Read the model definition and answer for the solid it produces. Units are mm, in the model's axes. Face numbers are marked on the shaded views. Coordinates: 2 decimals unless noted, no trailing zeros. Order: outer loops, then holes, each group sorted by start corner. A loop starts at its lowest first (then second) coordinate and runs counter-clockwise, first axis right, second up. Notation, with made-up numbers: (-37.5, -0.75) - (-11.5, -0.75) arc R11 cw to (-11.5, 5.25) - close; hole circle Ø9 at (44.5, 49.5). An arc over 180 degrees is marked (long way). Use one line per item in the form item = value.
```python
from build123d import *

# Parameters (mm, degrees)
F0_R      = 15.875
F1_DEPTH  = 3.175
F1_FACE_R = 15.875
F2_DEPTH  = 25.4
F2_TAPER  = 15
F3_R      = 8.5725
F4_DEPTH  = 25.4


with BuildPart() as f1:
    # F0 (on Top) → F1 (new body)
    with BuildSketch(Plane.XY):
        Circle(F0_R)
    extrude(amount=F1_DEPTH)

    # F1_face (on face) → F2 (join)
    with BuildSketch(Plane.XY.offset(3.175)):
        Circle(F1_FACE_R)
    extrude(amount=F2_DEPTH, taper=F2_TAPER)

    # F3 (on face) → F4 (cut)
    with BuildSketch(Plane.XY.offset(28.575)):
        Circle(F3_R)
    extrude(amount=-F4_DEPTH, mode=Mode.SUBTRACT)


solid = f1.part
```
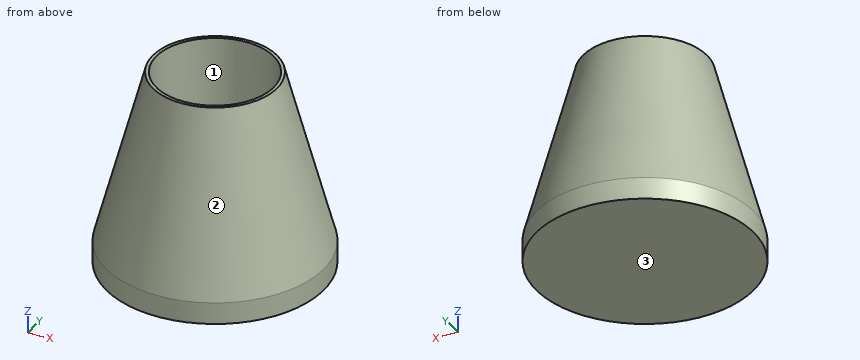
(1) The mould has two halves that part along X. Classify the marked faces 1, 2 and 3: +X half, -X half, draft (parallel to the pull), parting line (faces both ways), or undercut.
Answer list:
face_1 = undercut
face_2 = parting line
face_3 = draft
(2) Section D-D, the plane z = 12 is taken. Write down the section's boundary in (x, y) (1 decimal).
Answer list:
outline = circle Ø27 at (0, 0); hole circle Ø17.1 at (0, 0)
(3) Straight lines are drawn through the part: L1, parallel to Z at x = -4.5, y = 1.5 (3 decimals); L2, parallel to Y at x = 5, z = 21.5; L3, parallel to Y at x = 7.5, z = 12.5. For each, find the intervals that lie inside material, in ascending order.
Answer list:
L1 = 0 to 3.175
L2 = -9.76 to -6.96, 6.96 to 9.76
L3 = -11.08 to -4.15, 4.15 to 11.08
(4) Section C-C, the plane z = 24 is taken. Write down the section's boundary in (x, y) (1 decimal).
Answer list:
outline = circle Ø20.6 at (0, 0); hole circle Ø17.1 at (0, 0)
(5) Section A-A, the plane x = 0 is taken. Write down the section's boundary in (y, z) (1 decimal), then the cut area to 3 significant figures.
Answer list:
outline = (-15.9, 0) - (15.9, 0) - (15.9, 3.2) - (9.1, 28.6) - (8.6, 28.6) - (8.6, 3.2) - (-8.6, 3.2) - (-8.6, 28.6) - (-9.1, 28.6) - (-15.9, 3.2) - close
area = 299 mm2
(6) Given pin 1 Ø1 at (y, z) = (8, 4) entering from -X; pin 2 Ø5 at (x, y) = (-1, 0) entering from +Z (3 decimals); pin 3 Ø5 at (x, z) = (5, 13) entering from -Y, each flat-ended and moving along its own axis, determine where each tip first touches the part or whether it passes through.
Answer list:
pin_1 = -13.78
pin_2 = 3.175
pin_3 = -13.33
